Could you check a few things on this drawing? It's one solid part, dimensions in mm from its lowest x, y, z. A direction names the side the tool comes from. Round coordinates to 2 decimals unless told otherwise and drop trailing zeros. Write each loop counter-clockwise with the first axis right and the second up, starting at its lowest first coordinate (ties: lowest second). Pieces come first, ordered by that corner, then holes. Notation, with made-up numbers: (52, 11.25) -> (90, 11.25) arc R20 cw to (90, 48.25) -> close; hole circle Ø11 at (74.5, 29.5). An arc over 180 degrees is marked (long way). Return JSON: item names as keys, results as strings.
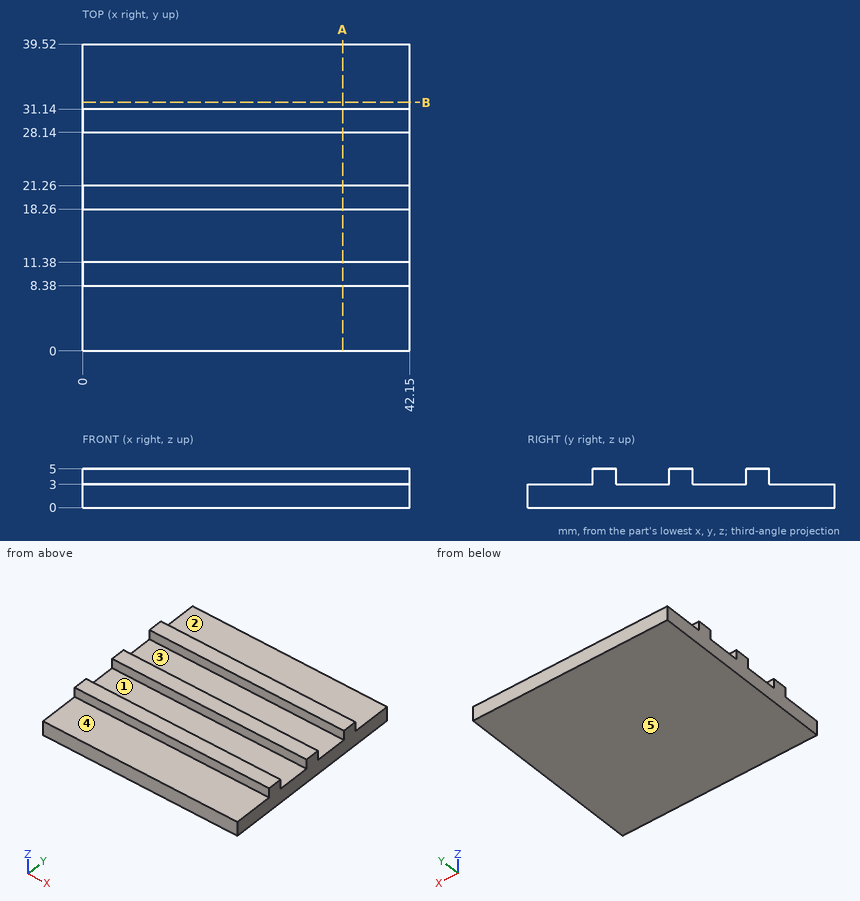
1) I want a section at A-A, the plane x = 33.5. Please give me the cut outline in (y, z).
Return value:
{"outline": "(0, 0) -> (39.52, 0) -> (39.52, 3) -> (31.14, 3) -> (31.14, 5) -> (28.14, 5) -> (28.14, 3) -> (21.26, 3) -> (21.26, 5) -> (18.26, 5) -> (18.26, 3) -> (11.38, 3) -> (11.38, 5) -> (8.38, 5) -> (8.38, 3) -> (0, 3) -> close"}
2) Will these pins go through, and if not, where does the flat tip stop? pin 1 Ø4 at (x, y) = (30.5, 5.5) entering from +Z; pin 2 Ø0.6 at (x, z) = (21.5, 4) entering from +Y; pin 3 Ø0.6 at (x, z) = (12.5, 4) entering from -Y.
Return value:
{"pin 1": "z = 3", "pin 2": "y = 31.14", "pin 3": "y = 8.38"}
3) Thinking about a two-plate mould opening in Y: for the marked faces 1 and 2, which applies, pulls with the +Y half, pulls with the -Y half, needs draft (parallel to the pull), parting line crosses it, or undercut?
Return value:
{"face 1": "undercut", "face 2": "needs draft"}
4) For the marked faces 3, 4 and 5, which set-ups out of +Z, -Z, +X, -X, +Y, -Y let a thin tool reach every point of the face, with its end or its side?
Return value:
{"face 3": "+Z, +X, -X", "face 4": "+Z, +X, -X, -Y", "face 5": "-Z, +X, -X, +Y, -Y"}
5) If I drill on probe 1 along Y at (x, z) = (24.5, 4.85); probe 2 along Z at (x, y) = (7, 31.5), over which ranges is the centre line in solid material (lowest first)? Write a range as [from, to].
Return value:
{"probe 1": "[8.38, 11.38], [18.26, 21.26], [28.14, 31.14]", "probe 2": "[0, 3]"}
6) I want a section at B-B, the plane y = 32. Please give me the cut outline in (x, z), and give its area (3 significant figures).
Return value:
{"outline": "(0, 0) -> (42.15, 0) -> (42.15, 3) -> (0, 3) -> close", "area": "126 mm²"}
